from build123d import *

# Parameters (mm, degrees)
SKETCH1_R                = 6
SKETCH1_R_2              = 5.3
BOSS_EXTRUDE1_DEPTH      = 11.2
SKETCH2_W                = 12
SKETCH2_H                = 12
BOSS_EXTRUDE2_DEPTH      = 1.6
SKETCH3_W                = 17.5
SKETCH3_H                = 12
BOSS_EXTRUDE3_DEPTH      = 6
CUT_EXTRUDE1_DEPTH       = 2.75
CIRPATTERN8_COUNT        = 2
SKETCH5_OUTSIDE_W        = 25.17
SKETCH5_OUTSIDE_H        = 19.67
SKETCH5_OUTSIDE_R        = 8.75
CUT_EXTRUDE2_DEPTH       = 22.587091205
BOSS_EXTRUDE4_DEPTH      = 5
SKETCH7_W                = 1.4
SKETCH7_H                = 2
BOSS_EXTRUDE5_DEPTH      = 5
SKETCH8_W                = 2.1
SKETCH8_H                = 27.5
BOSS_EXTRUDE6_DEPTH      = 15.7
CUT_EXTRUDE3_DEPTH       = 3
FILLET1_R                = 1
BOSS_EXTRUDE7_DEPTH      = 3.35
SKETCH12_W               = 2.9
SKETCH12_H               = 1.2
CUT_EXTRUDE4_DEPTH       = 6.7
CHAMFER1_SIZE            = 1
CHAMFER2_SIZE            = 2
SKETCH13_R               = 1.5
CUT_EXTRUDE5_DEPTH       = 6.7
CHAMFER1_OF_MIRROR3_SIZE = 1
CHAMFER2_OF_MIRROR3_SIZE = 2
SKETCH14_R               = 1.65
BOSS_EXTRUDE8_DEPTH      = 2


# Some blends are built 0.0001 mm under size
with BuildPart() as part:
    # Sketch1 → Boss-Extrude1 (new body)
    with BuildSketch(Plane(origin=(0, 0, 0), x_dir=(1, 0, 0), z_dir=(0, 1, 0))):
        with Locations(Location((0, 0, 0), (0, 0, 270))):
            Circle(SKETCH1_R)
        with Locations(Location((0, 0, 0), (0, 0, 270))):
            Circle(SKETCH1_R_2, mode=Mode.SUBTRACT)
    extrude(amount=BOSS_EXTRUDE1_DEPTH)

    # Sketch2 → Boss-Extrude2 (add)
    with BuildSketch(Plane.XZ):
        Rectangle(SKETCH2_W, SKETCH2_H)
    extrude(amount=BOSS_EXTRUDE2_DEPTH)

    # Sketch3 → Boss-Extrude3 (add)
    with BuildSketch(Plane.XZ.offset(1.6)):
        Rectangle(SKETCH3_W, SKETCH3_H)
    extrude(amount=BOSS_EXTRUDE3_DEPTH)

    # Sketch4 → Cut-Extrude1 (cut)
    with BuildSketch(Plane.ZY.offset(8.75)):
        with BuildLine():
            Line((3.5, -1.6), (3.5, -5.1))
            Line((3.5, -5.1), (-3.5, -5.1))
            Line((-3.5, -5.1), (-3.5, -4.6))
            add(Edge.make_bspline(
                [(-3.5, -4.6), (-3.5, -3.681946605), (-2.636311327, -2.93147779), (-0.605865115, -3.976002744), (0, -3.206492633), (0, -2.1)],
                knots=[0, 0, 0, 0, 0.306820438, 0.673720389, 1, 1, 1, 1], degree=3))
            Line((0, -2.1), (0, -1.6))
            Line((0, -1.6), (3.5, -1.6))
        make_face()
    cut_extrude1 = extrude(amount=-CUT_EXTRUDE1_DEPTH, mode=Mode.SUBTRACT)

    # CirPattern8: Cut-Extrude1 ×2 about axis
    cirpattern8_axis = Axis((0, 11.2, 0), (0, -1, 0))
    for i in range(1, CIRPATTERN8_COUNT):
        add(cut_extrude1.rotate(cirpattern8_axis, i * 360 / CIRPATTERN8_COUNT), mode=Mode.SUBTRACT)

    # Sketch5 outside → Cut-Extrude2 (cut, through all)
    with BuildSketch(Plane(origin=(0, 11.2, 0), x_dir=(1, 0, 0), z_dir=(0, 1, 0))):
        Rectangle(SKETCH5_OUTSIDE_W, SKETCH5_OUTSIDE_H)
        Circle(SKETCH5_OUTSIDE_R, mode=Mode.SUBTRACT)
    extrude(amount=-CUT_EXTRUDE2_DEPTH, mode=Mode.SUBTRACT)

    # Sketch6 → Boss-Extrude4 (add)
    with BuildSketch(Plane.XZ.offset(7.6)):
        Polygon((-6.168869601, -4.35), (-6.168869601, 4.35), (-7.768869601, 3), (-7.768869601, -3), align=None)
        Polygon((-4.768869601, -6), (-4.768869601, 6), (-6.168869601, 6), (-6.168869601, 4.35), (-6.168869601, -4.35), (-6.168869601, -6), align=None)
    extrude(amount=BOSS_EXTRUDE4_DEPTH)

    # Sketch7 → Boss-Extrude5 (add)
    with BuildSketch(Plane.XZ.offset(12.6)):
        with Locations((-5.468869601, 5)):
            Rectangle(SKETCH7_W, SKETCH7_H)
        with Locations((-5.468869601, -5)):
            Rectangle(SKETCH7_W, SKETCH7_H)
    extrude(amount=BOSS_EXTRUDE5_DEPTH)

    # Sketch8 → Boss-Extrude6 (add)
    with BuildSketch(Plane.XZ.offset(7.6)):
        with Locations((5.781130399, 0)):
            Rectangle(SKETCH8_W, SKETCH8_H)
    extrude(amount=BOSS_EXTRUDE6_DEPTH)

    # Sketch9 → Cut-Extrude3 (cut)
    with BuildSketch(Plane(origin=(6.831130399, 0, 0), x_dir=(0, 0, -1), z_dir=(1, 0, 0))):
        Polygon((-6.35, -23.3), (-5.25, -12.8), (5.55, -12.8), (7.25, -17.3), (13.75, -17.3), (13.75, -23.3), align=None)
    extrude(amount=-CUT_EXTRUDE3_DEPTH, mode=Mode.SUBTRACT)

    # Fillet1
    fillet1_edges = [part.edges().sort_by_distance(p)[0] for p in [
        (5.781130399, -7.6, 13.75),
        (5.781130399, -7.6, -13.75),
        (-5.468869601, -17.6, -6),
        (-5.468869601, -17.6, -4),
        (-5.468869601, -17.6, 6),
        (-5.468869601, -17.6, 4),
        (5.781130399, -23.3, 13.75),
        (5.781130399, -23.3, 6.35),
        (5.781130399, -17.3, -7.25),
        (5.781130399, -17.3, -13.75),
    ]]
    fillet(fillet1_edges, radius=FILLET1_R - 0.0001)  # a hair under: the kernel refuses the full size

    # Sketch11 → Boss-Extrude7 (add, symmetric)
    with BuildSketch(Plane.XY):
        Polygon((-6.168869601, -12.6), (-6.168869601, -15.599847371), (-8.268869601, -17.599847371), (-8.268869601, -25.599847371), (-7.768869601, -25.599847371), (-7.768869601, -17.814133086), (-5.668869601, -15.814133086), (-5.668869601, -12.6), align=None)
    boss_extrude7 = extrude(amount=BOSS_EXTRUDE7_DEPTH, both=True)

    # Sketch12 → Cut-Extrude4 (cut)
    with BuildSketch(Plane(origin=(4.856585084, -5.099414338, 0), x_dir=(0.7241379310344822, 0.6896551724137937, 0), z_dir=(-0.6896551724137937, 0.7241379310344822, 0))):
        with Locations((-16.675627899, 2.75)):
            Rectangle(SKETCH12_W, SKETCH12_H)
        with Locations((-16.675627899, -2.75)):
            Rectangle(SKETCH12_W, SKETCH12_H)
    cut_extrude4 = extrude(amount=-CUT_EXTRUDE4_DEPTH, mode=Mode.SUBTRACT)

    # Chamfer1
    # the kernel refuses this chamfer: 1 mm, written as the material it takes off along each edge
    with BuildSketch(Plane(origin=(-10.042444076, -15.737594173, -3.35), x_dir=(0.019910807200768887, 0.018962673524541826, 0.9996219169112968), z_dir=(0.6896551724137937, -0.7241379310344822, 0))) as chamfer1_piece_1:
        Polygon((CHAMFER1_SIZE * 0.999621916911, CHAMFER1_SIZE * 0.0274958766106), (-CHAMFER1_SIZE * 0.0274958766106, CHAMFER1_SIZE * 0.999621916911), (0, 0), align=None)
    extrude(amount=5.868365976, mode=Mode.SUBTRACT)
    with BuildSketch(Plane(origin=(-10.042444076, -15.737594173, 3.35), x_dir=(0.019910807200768887, 0.018962673524541826, -0.9996219169112968), z_dir=(0.6896551724137937, -0.7241379310344822, 0))) as chamfer1_piece_2:
        Polygon((CHAMFER1_SIZE * 0.999621916911, -CHAMFER1_SIZE * 0.0274958766106), (-CHAMFER1_SIZE * 0.0274958766106, -CHAMFER1_SIZE * 0.999621916911), (0, 0), align=None)
    extrude(amount=5.868365976, mode=Mode.SUBTRACT)

    # Chamfer2
    chamfer2_edges = [part.edges().sort_by_distance(p)[0] for p in [
        (-8.018869601, -25.599847371, -3.35),
        (-8.018869601, -25.599847371, 3.35),
    ]]
    chamfer(chamfer2_edges, length=CHAMFER2_SIZE)

    # Sketch13 → Cut-Extrude5 (cut)
    with BuildSketch(Plane.ZY.offset(8.268869601)):
        with Locations((0, -21.324847371)):
            Circle(SKETCH13_R)
    cut_extrude5 = extrude(amount=-CUT_EXTRUDE5_DEPTH, mode=Mode.SUBTRACT)

    # Mirror3: Boss-Extrude7, Cut-Extrude4, Cut-Extrude5 across plane
    add(boss_extrude7.mirror(Plane(origin=(0, 0, 0), x_dir=(0, 0, 1), z_dir=(1, 0, 0))))
    add(cut_extrude4.mirror(Plane(origin=(0, 0, 0), x_dir=(0, 0, 1), z_dir=(1, 0, 0))), mode=Mode.SUBTRACT)
    add(cut_extrude5.mirror(Plane(origin=(0, 0, 0), x_dir=(0, 0, 1), z_dir=(1, 0, 0))), mode=Mode.SUBTRACT)

    # Chamfer1 of Mirror3
    # the kernel refuses this chamfer: 1 mm, written as the material it takes off along each edge
    with BuildSketch(Plane(origin=(10.042444076, -15.737594173, -3.35), x_dir=(0.7238641467288695, -0.6893944254560673, -0.02749587661058651), z_dir=(-0.6896551724137937, -0.7241379310344822, 0))) as chamfer1_of_mirror3_piece_1:
        Polygon((CHAMFER1_OF_MIRROR3_SIZE * 0.999621916911, CHAMFER1_OF_MIRROR3_SIZE * 0.0274958766106), (-CHAMFER1_OF_MIRROR3_SIZE * 0.0274958766106, CHAMFER1_OF_MIRROR3_SIZE * 0.999621916911), (0, 0), align=None)
    extrude(amount=5.868365976, mode=Mode.SUBTRACT)
    with BuildSketch(Plane(origin=(10.042444076, -15.737594173, 3.35), x_dir=(0.7238641467288695, -0.6893944254560673, 0.02749587661058651), z_dir=(-0.6896551724137937, -0.7241379310344822, 0))) as chamfer1_of_mirror3_piece_2:
        Polygon((CHAMFER1_OF_MIRROR3_SIZE * 0.999621916911, -CHAMFER1_OF_MIRROR3_SIZE * 0.0274958766106), (-CHAMFER1_OF_MIRROR3_SIZE * 0.0274958766106, -CHAMFER1_OF_MIRROR3_SIZE * 0.999621916911), (0, 0), align=None)
    extrude(amount=5.868365976, mode=Mode.SUBTRACT)

    # Chamfer2 of Mirror3
    chamfer2_of_mirror3_edges = [part.edges().sort_by_distance(p)[0] for p in [
        (8.018869601, -25.599847371, -3.35),
        (8.018869601, -25.599847371, 3.35),
    ]]
    chamfer(chamfer2_of_mirror3_edges, length=CHAMFER2_OF_MIRROR3_SIZE)

    # Sketch14 → Boss-Extrude8 (add)
    with BuildSketch(Plane.ZY.offset(-4.731130399)):
        with Locations(Location((-11.25, -10.3, 0), (0, 0, 180))):
            Circle(SKETCH14_R)
        with Locations(Location((10.95, -20.6, 0), (0, 0, 180))):
            Circle(SKETCH14_R)
    extrude(amount=BOSS_EXTRUDE8_DEPTH)


solid = part.part
Geometry check sheet. Reference: the model listing, model coordinates, mm. A direction names the side the tool comes from. Round coordinates to 2 decimals unless told otherwise and drop trailing zeros. Order: outer loops, then holes, each group sorted by start corner. A loop starts at its lowest first (then second) coordinate and runs counter-clockwise, first axis right, second up. Notation, with made-up numbers: (47, 56) - (98, 56) arc R7 cw to (98, 65) - close; hole circle Ø1 at (-20.75, 33). An arc over 180 degrees is marked (long way). One line per question, with ' | ' between items. Start each with the question number.
(1) Release check for a two-part mould opening along Z. For faces 1 (the flat face through (0, -4, -6)), 2 (the cylindrical face through (8.02, -22.79, -0.33)), 3 (the flat face through (-8, -7.6, 0)) record: released by +Z, released by -Z, zero draft, split by the parting line, or undercut.
(2) Sectioned sample at C-C on z = 10.95. Record the cut outline in (x, y).
(3) Access from +Z, -Z, +X, -X, +Y, -Y to the whole of each face (thin tool, end or side, straight path). Record for faces 4 (the flat face through (5, 0, 5)), 5 (the cylindrical face through (-5.459, -17.315, -4.301)), 6 (the flat face through (8, -7.6, 0)), 7 (the flat face through (7, -5.1, 0)).
(4) Thickness scan on L1, parallel to X at y = 5.5, z = 0; L2, parallel to Y at x = -1.25, z = 2.5; L3, parallel to X at y = -15, z = 10.75. Record the ranges inside material, lowest first. Write a range as [from, to].
(5) Sectioned sample at B-B on z = -11.25. Record the cut outline in (x, y), and give its area (3 significant figures).
(6) Sectioned sample at A-A on y = -10.3. Record the cut outline in (x, z), and give its area (3 significant figures).
(7) Sectioned sample at D-D on x = -1.5. Record the cut outline in (y, z).
(8) Depth check by flat-ended pin: pin 1 Ø1.7 at (x, z) = (6, -11.5) entering from -Y; pin 2 Ø3 at (y, z) = (-14.5, 8.5) entering from -X; pin 3 Ø0.7 at (x, y) = (-5, -14.5) entering from -Z. Enter the tip coordinate at first touch or a pass-through.
Conclusion:
1) face 1: released by -Z | face 2: undercut | face 3: zero draft
2) outline: (2.73, -22.25) - (4.73, -22.25) - (4.73, -23.3) - (6.83, -23.3) - (6.83, -7.6) - (4.73, -7.6) - (4.73, -18.95) - (2.73, -18.95) - close
3) face 4: +Z, +X, +Y | face 5: +X, -X, -Y | face 6: +Z, -Z, +X | face 7: +X
4) L1: x = [-6, -5.3], [5.3, 6] | L2: y = [-7.6, 0] | L3: x = [4.73, 6.83]
5) outline: (2.73, -11.95) - (4.73, -11.95) - (4.73, -17.3) - (6.83, -17.3) - (6.83, -7.6) - (4.73, -7.6) - (4.73, -8.65) - (2.73, -8.65) - close | area: 27.0 mm2
6) outline: (-7.77, -3) - (-6.17, -4.35) - (-6.17, -6) - (-4.77, -6) - (-4.77, 6) - (-6.17, 6) - (-6.17, 4.35) - (-7.77, 3) - close; (2.73, -12.9) - (4.73, -12.9) - (4.73, -13.75) - (6.83, -13.75) - (6.83, 13.75) - (4.73, 13.75) - (4.73, -9.6) - (2.73, -9.6) - close | area: 92.9 mm2
7) outline: (-7.6, -6) - (0, -6) - (0, -5.81) - (11.2, -5.81) - (11.2, -5.08) - (0, -5.08) - (0, 5.08) - (11.2, 5.08) - (11.2, 5.81) - (0, 5.81) - (0, 6) - (-7.6, 6) - close
8) pin 1: stops at y = -17.3 | pin 2: stops at x = 4.73 | pin 3: stops at z = -6
